Geometry: final body of the model. Coordinates: model frame, mm. Give positions to 0.01 mm unless a question says otherwise; leave off trailing zeros. Loops run counter-clockwise (first coordinate to the right, second up) from the corner with the lowest first, then second, coordinate; pieces in that order, holes last. Notation, with made-up numbers: (65.25, 28.25) - (75.25, 28.25) arc R20 ccw to (75.25, 39.25) - close; hole circle Ø11 at (-26.5, 55.5). An arc over 180 degrees is marked (long way). Use CSV: the item, a comma, the result in double quotes. Start each with the question number.
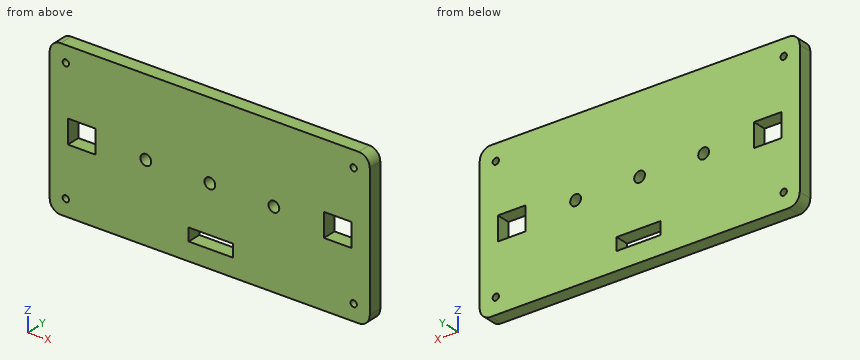
```python
from build123d import *

# Parameters (mm, degrees)
SKETCH1_W           = 147.828
SKETCH1_H           = 71.501
BOSS_EXTRUDE1_DEPTH = 6.35
FILLET1_R           = 5.08
SKETCH2_R           = 2.4892
SKETCH2_W           = 12.7508
SKETCH2_H           = 10.8712
CUT_EXTRUDE1_DEPTH  = 7.35
SKETCH3_R           = 1.4605
CUT_EXTRUDE2_DEPTH  = 7.35
SKETCH5_W           = 20.391623785
SKETCH5_H           = 5.837943421
CUT_EXTRUDE3_DEPTH  = 7.35


with BuildPart() as part:
    # Sketch1 → Boss-Extrude1 (new body)
    with BuildSketch(Plane(origin=(0, 0, 0), x_dir=(1, 0, 0), z_dir=(0, 1, 0))):
        Rectangle(SKETCH1_W, SKETCH1_H)
    extrude(amount=BOSS_EXTRUDE1_DEPTH)

    # Fillet1
    fillet1_edges = [part.edges().sort_by_distance(p)[0] for p in [
        (73.914, 3.175, 35.7505),
        (-73.914, 3.175, 35.7505),
        (-73.914, 3.175, -35.7505),
        (73.914, 3.175, -35.7505),
    ]]
    fillet(fillet1_edges, radius=FILLET1_R)

    # Sketch2 → Cut-Extrude1 (cut, through all)
    with BuildSketch(Plane(origin=(0, 6.35, 0), x_dir=(1, 0, 0), z_dir=(0, 1, 0))):
        with Locations((-29.505731413, 0)):
            Circle(SKETCH2_R)
        with Locations((29.625468587, 0)):
            Circle(SKETCH2_R)
        with Locations((0.059868587, 0)):
            Circle(SKETCH2_R)
        with Locations((59.1312, 0)):
            Rectangle(SKETCH2_W, SKETCH2_H)
        with Locations((-59.1312, 0)):
            Rectangle(SKETCH2_W, SKETCH2_H)
    extrude(amount=-CUT_EXTRUDE1_DEPTH, mode=Mode.SUBTRACT)

    # Sketch3 → Cut-Extrude2 (cut, through all)
    with BuildSketch(Plane(origin=(0, 6.35, 0), x_dir=(1, 0, 0), z_dir=(0, 1, 0))):
        with Locations((-66.4845, 28.321)):
            Circle(SKETCH3_R)
        with Locations((66.4845, 28.321)):
            Circle(SKETCH3_R)
        with Locations((66.4845, -28.321)):
            Circle(SKETCH3_R)
        with Locations((-66.4845, -28.321)):
            Circle(SKETCH3_R)
    extrude(amount=-CUT_EXTRUDE2_DEPTH, mode=Mode.SUBTRACT)

    # Sketch5 → Cut-Extrude3 (cut, through all)
    with BuildSketch(Plane(origin=(0, 6.35, 0), x_dir=(1, 0, 0), z_dir=(0, 1, 0))):
        with Locations((0.498877124, 24.544882744)):
            Rectangle(SKETCH5_W, SKETCH5_H)
    extrude(amount=-CUT_EXTRUDE3_DEPTH, mode=Mode.SUBTRACT)


solid = part.part
```
Item 1: Section C-C (z = 0). Output: boundary loops of the cut face in (x, y), plus the area to 3 significant figures.
Item 2: Pin query (flat end, axial travel): pin 1 Ø5.5 at (x, z) = (29.63, 0) entering from -Y. Return the tip coordinate at first contact, or that it passes through.
Item 3: Section A-A (x = -62.5). Output: boundary loops of the cut face in (y, z), plus the area to 3 significant figures.
Item 4: Section B-B (z = -23.5). Output: boundary loops of the cut face in (x, y), plus the area to 3 significant figures.
Item 5: Ray query, probe 1 along X at (y, z) = (2, 0); probe 2 along X at (y, z) = (4, 4); probe 3 along X at (y, z) = (5, 28.5). Return the intervals inside material, ascending.
Item 6: Section D-D (y = 3.75). Give the number of separate pieces and of enclosed holes in the cut face, plus the area to 3 significant figures.
Outcome:
1,outline,"(-73.91, 0) - (-65.51, 0) - (-65.51, 6.35) - (-73.91, 6.35) - close; (-52.76, 0) - (-31.99, 0) - (-31.99, 6.35) - (-52.76, 6.35) - close; (-27.02, 0) - (-2.43, 0) - (-2.43, 6.35) - (-27.02, 6.35) - close; (2.55, 0) - (27.14, 0) - (27.14, 6.35) - (2.55, 6.35) - close; (32.11, 0) - (52.76, 0) - (52.76, 6.35) - (32.11, 6.35) - close; (65.51, 0) - (73.91, 0) - (73.91, 6.35) - (65.51, 6.35) - close"
1,area,"682 mm2"
2,pin 1,"stops at y = 0"
3,outline,"(0, -35.75) - (6.35, -35.75) - (6.35, -5.44) - (0, -5.44) - close; (0, 5.44) - (6.35, 5.44) - (6.35, 35.75) - (0, 35.75) - close"
3,area,"385 mm2"
4,outline,"(-73.91, 0) - (-9.7, 0) - (-9.7, 6.35) - (-73.91, 6.35) - close; (10.69, 0) - (73.91, 0) - (73.91, 6.35) - (10.69, 6.35) - close"
4,area,"809 mm2"
5,probe 1,"x = -73.91 to -65.51, -52.76 to -31.99, -27.02 to -2.43, 2.55 to 27.14, 32.11 to 52.76, 65.51 to 73.91"
5,probe 2,"x = -73.91 to -65.51, -52.76 to 52.76, 65.51 to 73.91"
5,probe 3,"x = -73.91 to -67.93, -65.04 to 65.04, 67.93 to 73.91"
6,separate pieces,"1"
6,enclosed holes,"10"
6,area,"10,100 mm2"
